CAD build for the part. Positions are in the model's coordinates, mm. Face numbers are marked on the shaded views. A direction names the side the tool comes from. Give positions to 0.01 mm unless a question says otherwise; leave off trailing zeros. Order: outer loops, then holes, each group sorted by start corner. A loop starts at its lowest first (then second) coordinate and runs counter-clockwise, first axis right, second up. Notation, with made-up numbers: (-24.75, 38.5) -> (-17.75, 38.5) arc R27 ccw to (-17.75, 71.5) -> close; hole circle Ø2 at (69.25, -14.75). An arc over 180 degrees is marked (long way). Use one line per item in the form item = value. Start each with the question number.
1) Cut at C-C, the plane z = 44. Give the cut face in (x, y).
2) Cut at B-B, the plane y = 63.5. State how many separate pieces and enclosed holes the cut face has, and give its area (3 significant figures).
3) Mould opens along Z. For the marked faces 3, 4 and 5 say: pulls with the +Z half, pulls with the -Z half, needs draft (parallel to the pull), parting line crosses it, or undercut.
4) Cut at D-D, the plane x = 12.7. Give the cut face in (y, z), and give its area (3 significant figures).
5) Drop flat-ended pins along their axis: P1, Ø5.5, axis at y = 12.7, z = 12.73, coming from the +X side; P2, Ø1.3, axis at y = 27.5, z = -1, coming from the -X side. Give the stop position or say it passes through.
6) Tool access for the marked faces 1 and 2: list every direction of +Z, -Z, +X, -X, +Y, -Y with a clear straight run to the whole face (end or side of a thin tool).
7) Cut at A-A, the plane x = 57.5. Give the cut face in (y, z), and give its area (3 significant figures).
8) Probe line 1 (X direction, y = 36.5, z = 25.5); line 2 (Z direction, x = 9.5, y = 27.5); line 3 (Z direction, x = 78, y = 12). List the from-to ranges inside material, lowest first.
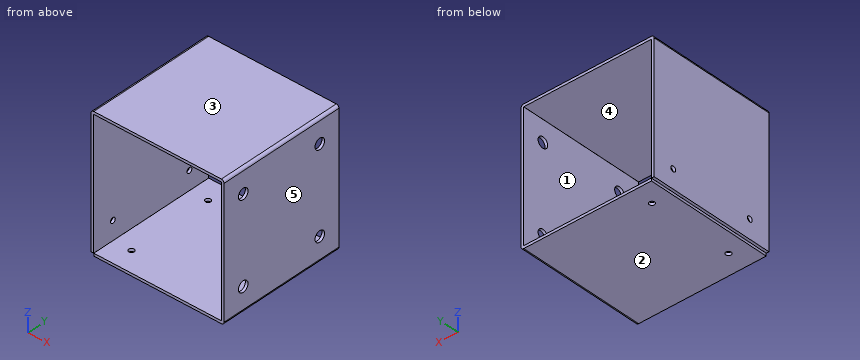
Autodesk Inventor part; units mm, degrees
ref_plane "YZ Plane" through (0, 0, 0) normal (1, 0, 0) x (0, 1, 0)
ref_plane "XZ Plane" through (0, 0, 0) normal (0, 1, 0) x (-1, 0, 0)
ref_plane "XY Plane" through (0, 0, 0) normal (0, 0, 1) x (1, 0, 0)
sketch "Sketch4" plane through (0, 0, 0) normal (1, 0, 0) x (0, 1, 0)
  line L0 (0, 0) -> (76.2, 0)
  line L1 (76.2, 0) -> (76.2, 304.8)
  line L2 (76.2, 304.8) -> (0, 304.8)
  line L3 (0, 304.8) -> (0, 0)
  dimension "d7" = 76.2
  dimension "d8" = 304.8
extrude "Extrusion2" add sketch "Sketch4" along normal blind 1.5875
sketch "Sketch5" plane through (1.5875, 0, 0) normal (1, 0, 0) x (0, 0, -1)
  line L0 (0, 0) -> (0, 76.2)
  line L1 (0, 76.2) -> (-304.8, 76.2)
  line L2 (-304.8, 76.2) -> (-304.8, 0)
  line L3 (-304.8, 0) -> (0, 0)
  line L4 (-228.6, 76.2) -> (-228.6, 0)
  line L5 (-152.4, 76.2) -> (-152.4, 0)
  line L6 (-76.2, 76.2) -> (-76.2, 0)
  dimension "d11" = 76.2
  dimension "d12" = 76.2
  dimension "d13" = 76.2
bend part "Bend Part2" radius 0.0162 angle 90 line through (1.5875, 76.2, 228.6) along (0, -1, 0) centre toward (1, 0, 0) moving side (0, 0, 1) both sides no
sketch "Sketch6" plane through (1.5875, 0, 0) normal (1, 0, 0) x (0, 0, -1)
  line L0 (-228.6, 0) -> (-228.6, 76.2)
  line L1 (-228.6, 0) -> (0, 0)
  line L2 (0, 76.2) -> (-228.6, 76.2)
  line L3 (-152.4, 76.2) -> (-152.4, 0)
  dimension "d16" = 76.2
bend part "Bend Part3" radius 0.0162 angle 90 line through (1.5875, 76.2, 152.4) along (0, -1, 0) centre toward (1, 0, 0) moving side (0, 0, 1) both sides no
sketch "Sketch7" plane through (1.5875, 0, 0) normal (1, 0, 0) x (0, 0, -1)
  line L0 (-152.4, 0) -> (-152.4, 76.2)
  line L1 (-152.4, 0) -> (0, 0)
  line L2 (0, 76.2) -> (-152.4, 76.2)
  line L3 (-76.2, 76.2) -> (-76.2, -0.6756)
  dimension "d19" = 76.2
bend part "Bend Part4" radius 0.0162 angle 90 line through (1.5875, 76.2, 76.2) along (0, -1, 0) centre toward (1, 0, 0) moving side (0, 0, 1) both sides no
sketch "Sketch8" plane through (77.7783, 0, -1.5783) normal (0, 0, -1) x (-1, 0, 0)
  line L0 (76.1746, 0) -> (0, 0)
  line L1 (0, 76.2) -> (76.1746, 76.2)
  line L2 (77.7783, 0) -> (77.7783, 76.2)
  point P0 (65.0783, 63.5)
  point P1 (65.0783, 12.7)
  dimension "d22" = 12.7
  dimension "d23" = 12.7
  dimension "d24" = 12.7
  dimension "d25" = 12.7
hole "Hole1" at (12.7, 63.5, -1.5783) at (12.7, 12.7, -1.5783) direction (0, 0, 1) diameter 3.175 depth 25.4 tip angle 118
sketch "Sketch9" plane through (0, 0, 0) normal (-1, 0, 0) x (0, 0, 1)
  line L0 (0, 76.2) -> (76.2, 76.2)
  line L1 (76.2, 0) -> (0, 0)
  line L2 (-1.5783, 76.2) -> (-1.5783, 0)
  point P0 (11.1217, 63.5)
  point P1 (11.1217, 12.7)
  dimension "d33" = 12.7
  dimension "d34" = 12.7
  dimension "d35" = 12.7
  dimension "d36" = 12.7
hole "Hole2" at (0, 63.5, 11.1217) at (0, 12.7, 11.1217) direction (1, 0, 0) diameter 3.175 depth 25.4 tip angle 118
sketch "Sketch10" plane through (79.3819, 0, 76.2) normal (1, 0, 0) x (0, 0, -1)
  line L0 (0, 76.2) -> (0, 0)
  line L1 (76.1746, 0) -> (0, 0)
  line L2 (76.1746, 76.2) -> (76.1746, 0)
  line L3 (0, 76.2) -> (76.1746, 76.2)
  point P0 (76.2, 0)
sketch "Sketch11" plane through (79.3819, 0, 76.2) normal (1, 0, 0) x (0, 0, -1)
  line L0 (76.1746, 76.2) -> (76.1746, 0)
  line L1 (0, 76.2) -> (76.1746, 76.2)
  line L2 (76.1746, 0) -> (0, 0)
  point P0 (76.2, 0)
  point P1 (12.6746, 63.5)
  point P2 (63.4746, 63.5)
  point P3 (12.6746, 12.7)
  point P4 (63.4746, 12.7)
  dimension "d46" = 12.7
  dimension "d47" = 12.7
  dimension "d49" = 12.7
  dimension "d57" = 12.7
  dimension "d58" = 12.7
  dimension "d59" = 50.8
  dimension "d60" = 50.8
  dimension "d61" = 12.7
hole "Hole3" at (79.3819, 63.5, 63.5254) at (79.3819, 63.5, 12.7254) at (79.3819, 12.7, 63.5254) at (79.3819, 12.7, 12.7254) direction (-1, 0, 0) diameter 6.35 depth 25.4 tip angle 118
properties part number "Box"
Result:
q1.outline = (0, 0) -> (1.59, 0) -> (1.59, 76.2) -> (0, 76.2) -> close; (77.79, 0) -> (79.38, 0) -> (79.38, 76.2) -> (77.79, 76.2) -> close
q2.separate_pieces = 5
q2.enclosed_holes = 0
q2.area = 460 mm²
q3.face_3 = pulls with the +Z half
q3.face_4 = undercut
q3.face_5 = needs draft
q4.outline = (0, -1.58) -> (11.11, -1.58) -> (11.11, 0.01) -> (0, 0.01) -> close; (0, 76.22) -> (76.2, 76.22) -> (76.2, 77.8) -> (0, 77.8) -> close; (14.29, -1.58) -> (61.91, -1.58) -> (61.91, 0.01) -> (14.29, 0.01) -> close; (65.09, -1.58) -> (76.2, -1.58) -> (76.2, 0.01) -> (65.09, 0.01) -> close
q4.area = 232 mm²
q5.P1 = 1.59
q5.P2 = 1.6
q6.face_1 = +Y, -Y
q6.face_2 = -Z, +X, -X, +Y, -Y
q7.outline = (0, -1.58) -> (76.2, -1.58) -> (76.2, 0.01) -> (0, 0.01) -> close; (0, 76.22) -> (76.2, 76.22) -> (76.2, 77.8) -> (0, 77.8) -> close
q7.area = 242 mm²
q8.line_1 = 0 to 1.59, 77.79 to 79.38
q8.line_2 = -1.58 to 0.01, 76.22 to 77.8
q8.line_3 = -1.56 to 9.63, 15.82 to 60.43, 66.62 to 77.79
